Can you work these out from the model? Positions are in its coordinate system, mm. Face numbers are marked on the shaded views. Coordinates: 2 decimals unless noted, no trailing zeros. Order: outer loops, then holes, each group sorted by start corner. A loop starts at its lowest first (then second) coordinate and runs counter-clockwise, first axis right, second up. Notation, with made-up numbers: (68.25, -38) - (96.25, -38) arc R27 cw to (96.25, -1) - close; hole circle Ø3 at (84, 26). An arc over 180 degrees is marked (long way). Return JSON: item names as keys, results as strings. Group by question number.
1) If we mould it in two halves opening along X, with no side actions, what happens to the marked faces 1, 2 and 3? For each: pulls with the +X half, pulls with the -X half, needs draft (parallel to the pull), parting line crosses it, or undercut.
2) Imagine slicing it at C-C (z = 1.5). Write out the boundary of the cut face in (x, y), and give its area (3 significant figures).
3) For pin 1 Ø4 at (x, z) = (-18.5, 10.5) entering from +Y; pin 2 Ø4 at (y, z) = (-3.5, 2) entering from -X; pin 3 Ø1 at (y, z) = (-9, 8) entering from -X, each with a flat end and sliding along its axis, tell me the tip position at first contact or that it passes through.
4) Imagine slicing it at A-A (y = 0). Write out the boundary of the cut face in (x, z), and give its area (3 significant figures).
5) If I drill on line 1 along Y through (x, z) = (0, 3.25); line 2 along X through (y, z) = (11, 5); line 3 along X through (y, z) = (-7, 6), over which ranges is the centre line in solid material (lowest first)?
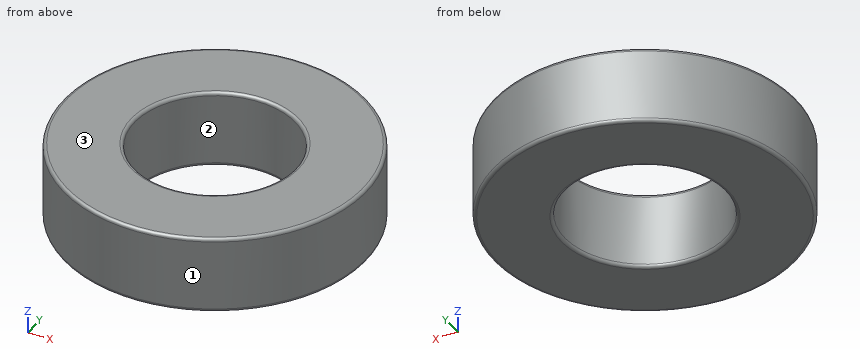
```python
from build123d import *

# Parameters (mm, degrees)
SKETCH1_R           = 23.5
SKETCH1_R_2         = 12.5
BOSS_EXTRUDE1_DEPTH = 12
FILLET1_R           = 0.5
FILLET2_R           = 0.5


with BuildPart() as part:
    # Sketch1 → Boss-Extrude1 (new body)
    with BuildSketch(Plane.XY):
        Circle(SKETCH1_R)
        Circle(SKETCH1_R_2, mode=Mode.SUBTRACT)
    extrude(amount=BOSS_EXTRUDE1_DEPTH)

    # Fillet1
    fillet1_edges = [part.edges().sort_by_distance(p)[0] for p in [
        (-23.5, 0, 0),
        (-23.5, 0, 12),
    ]]
    fillet(fillet1_edges, radius=FILLET1_R)

    # Fillet2
    fillet2_edges = [part.edges().sort_by_distance(p)[0] for p in [
        (-12.5, 0, 0),
        (-12.5, 0, 12),
    ]]
    fillet(fillet2_edges, radius=FILLET2_R)


solid = part.part
```
Calculated:
{
 "1": {"face 1": "parting line crosses it", "face 2": "undercut", "face 3": "needs draft"},
 "2": {"outline": "circle Ø47 at (0, 0); hole circle Ø25 at (0, 0)", "area": "1,240 mm2"},
 "3": {"pin 1": "y = 16.73", "pin 2": "x = -23.45", "pin 3": "x = -21.91"},
 "4": {"outline": "(-23.5, 0.5) arc R0.5 ccw to (-23, 0) - (-13, 0) arc R0.5 ccw to (-12.5, 0.5) - (-12.5, 11.5) arc R0.5 ccw to (-13, 12) - (-23, 12) arc R0.5 ccw to (-23.5, 11.5) - close; (12.5, 0.5) arc R0.5 ccw to (13, 0) - (23, 0) arc R0.5 ccw to (23.5, 0.5) - (23.5, 11.5) arc R0.5 ccw to (23, 12) - (13, 12) arc R0.5 ccw to (12.5, 11.5) - close", "area": "264 mm2"},
 "5": {"line 1": "-23.5 to -12.5, 12.5 to 23.5", "line 2": "-20.77 to -5.94, 5.94 to 20.77", "line 3": "-22.43 to -10.36, 10.36 to 22.43"}
}
